Source: three-view drawing plus pictorial views. Frame: mm from the lowest corner of the part. A direction names the side the tool comes from. Round coordinates to 2 decimals unless told otherwise and drop trailing zeros. Write each loop counter-clockwise with the first axis right and the second up, starting at its lowest first coordinate (ties: lowest second). Pieces come first, ordered by that corner, then holes. Notation, with made-up numbers: M -28,61.25 L 6,61.25 A29 cw 6,93.25 Z; hole C 54,70 d8. An arc over 180 degrees is marked long. Put each result on its own line as item: value. Start each with the question number.
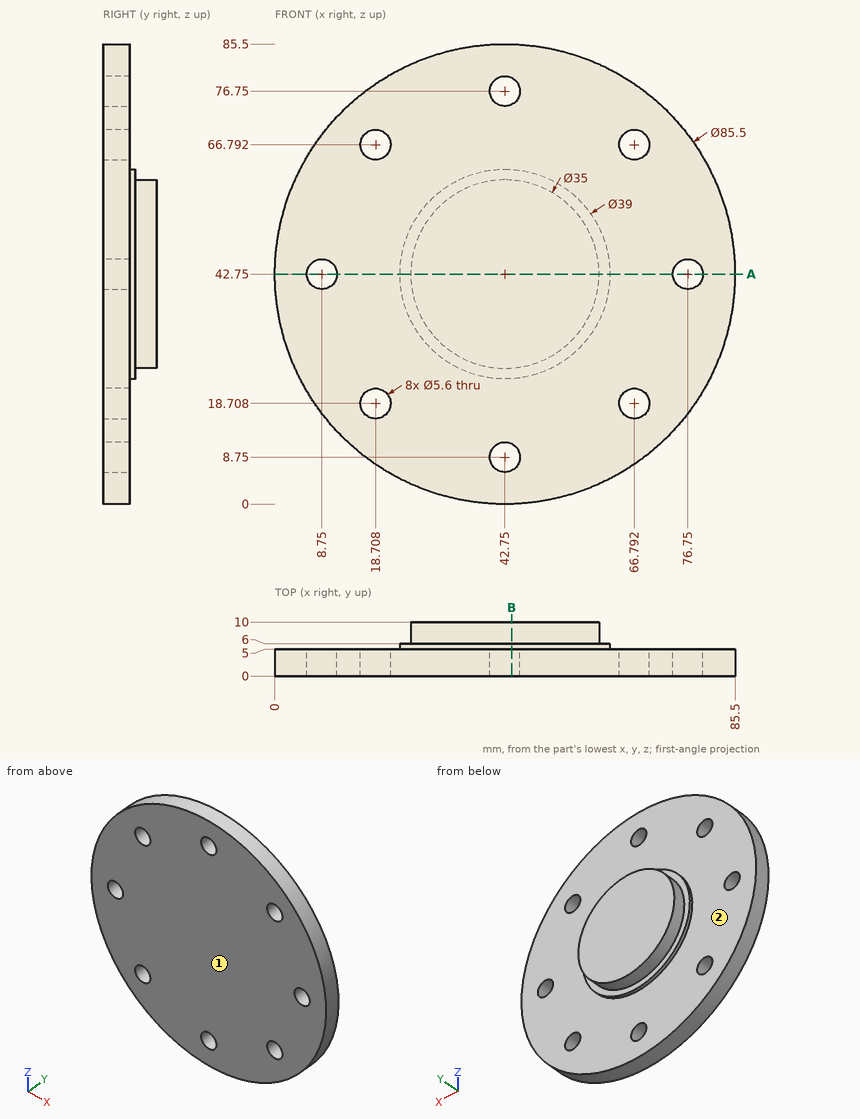
(1) Contact query for flat-ended pins moving along their axis: P1, Ø3, axis at x = 71.5, y = 3, coming from the -Z side; P2, Ø2, axis at y = 5, z = 68.5, coming from the +X side; P3, Ø6.5, axis at x = 42.75, z = 8.75, coming from the +Y side; P4, Ø3.5, axis at x = 76.75, z = 42.75, coming from the -Y side. Output: stop coordinate, or through.
(2) Section query A-A (z = 42.75). Return loops of the section in (x, y).
(3) Access query for the marked faces 1 and 2. Directions: +Z, -Z, +X, -X, +Y, -Y. A direction counts if a zero-diameter tool reaches every point of the face in a straight line with its end or side. Return the directions, or none.
(4) Section query B-B (x = 44). Return loops of the section in (y, z) (1 decimal).
(5) Ray query, line 1 along X through (y, z) = (4, 45) (1 decimal); line 2 along Y through (x, z) = (56.5, 69.5); line 3 along X through (y, z) = (2.75, 76). Return the intervals inside material, ascending.
Entries:
1. P1: z = 9.81
1. P2: x = 77.61
1. P3: y = 5
1. P4: through
2. outline: M 0,0 L 5.95,0 L 5.95,5 L 0,5 Z; M 11.55,0 L 73.95,0 L 73.95,5 L 62.25,5 L 62.25,6 L 60.25,6 L 60.25,10 L 25.25,10 L 25.25,6 L 23.25,6 L 23.25,5 L 11.55,5 Z; M 79.55,0 L 85.5,0 L 85.5,5 L 79.55,5 Z
3. face 1: +Z, -Z, +X, -X, -Y
3. face 2: +Y
4. outline: M 0,0 L 5,0 L 5,6.2 L 0,6.2 Z; M 0,11.3 L 5,11.3 L 5,23.3 L 6,23.3 L 6,25.3 L 10,25.3 L 10,60.2 L 6,60.2 L 6,62.2 L 5,62.2 L 5,74.2 L 0,74.2 Z; M 0,79.3 L 5,79.3 L 5,85.5 L 0,85.5 Z
5. line 1: 0.1 to 7.1, 10.4 to 75.1, 78.4 to 85.4
5. line 2: 0 to 5
5. line 3: 15.88 to 40.05, 45.45 to 69.62
